Input: dimensioned drawing with shaded views. Units: mm. Origin: part minimum x, y, z. A direction names the side the tool comes from. Coordinates: 2 decimals unless noted, no trailing zeros. Order: outer loops, then holes, each group sorted by start corner. A loop starts at its lowest first (then second) coordinate and runs counter-clockwise, first axis right, second up. Notation, with made-up numbers: (69.25, 32.25) - (106.25, 32.25) arc R20 cw to (106.25, 42.25) - close; hole circle Ø2 at (26.5, 30). An arc over 180 degrees is marked (long way). One line per question, with ' | ' between items. Start each with the question number.
(1) Access query for the marked faces 1, 2, 3 and 4. Directions: +Z, -Z, +X, -X, +Y, -Y. A direction counts if a zero-diameter tool reaches every point of the face in a straight line with its end or side. Return the directions, or none.
(2) Section B-B (x = 9.5). Return the cut outline in (y, z) (1 decimal).
(3) Section A-A (y = 6). Return the cut outline in (x, z).
(4) Section D-D (y = 2.5). Return the cut outline in (x, z).
(5) Line query: line 1 along X through (y, z) = (6.5, 0.4); line 2 along Y through (x, z) = (11.47, 2.75); line 3 along X through (y, z) = (9.5, 2.75). Output: solid intervals per line, ascending.
(6) Section C-C (z = 1.3). Return the cut outline in (x, y), then the cut area to 3 significant figures.
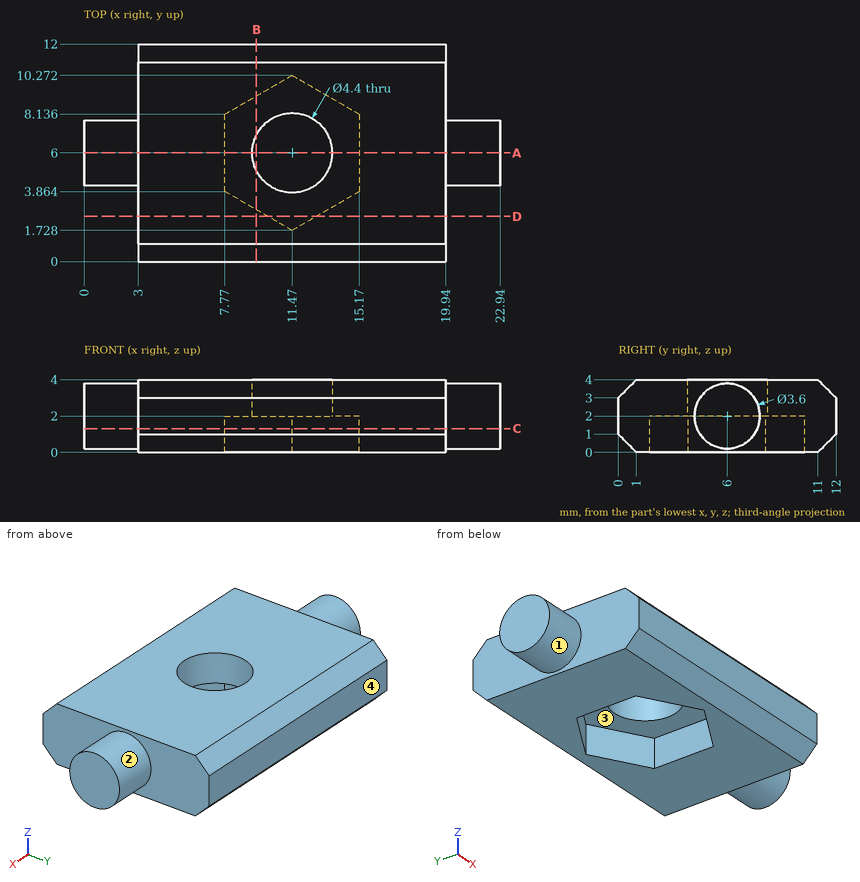
Response values:
1) face 1: -X | face 2: +X | face 3: -Z | face 4: +Z, -Z, +X, -X, +Y
2) outline: (0, 1) - (1, 0) - (2.9, 0) - (2.9, 2) - (5, 2) - (5, 4) - (1, 4) - (0, 3) - close; (7, 2) - (9.1, 2) - (9.1, 0) - (11, 0) - (12, 1) - (12, 3) - (11, 4) - (7, 4) - close
3) outline: (0, 0.2) - (3, 0.2) - (3, 0) - (7.77, 0) - (7.77, 2) - (9.27, 2) - (9.27, 4) - (3, 4) - (3, 3.8) - (0, 3.8) - close; (13.67, 2) - (15.17, 2) - (15.17, 0) - (19.94, 0) - (19.94, 0.2) - (22.94, 0.2) - (22.94, 3.8) - (19.94, 3.8) - (19.94, 4) - (13.67, 4) - close
4) outline: (3, 0) - (10.13, 0) - (10.13, 2) - (12.81, 2) - (12.81, 0) - (19.94, 0) - (19.94, 4) - (3, 4) - close
5) line 1: x = 0 to 7.77, 15.17 to 22.94 | line 2: y = 0 to 3.8, 8.2 to 12 | line 3: x = 3 to 19.94
6) outline: (0, 4.34) - (3, 4.34) - (3, 0) - (19.94, 0) - (19.94, 4.34) - (22.94, 4.34) - (22.94, 7.66) - (19.94, 7.66) - (19.94, 12) - (3, 12) - (3, 7.66) - (0, 7.66) - close; hole (7.77, 3.86) - (11.47, 1.73) - (15.17, 3.86) - (15.17, 8.14) - (11.47, 10.27) - (7.77, 8.14) - close | area: 176 mm²
